Geometry: final body of the model. Coordinates: model frame, mm. A direction names the side the tool comes from. Give positions to 0.01 mm unless a question says otherwise; leave off trailing zeros. Write each loop counter-clockwise with the first axis right and the second up, starting at its lowest first coordinate (ties: lowest second). Pieces come first, ordered by that corner, then holes. Notation, with made-up numbers: (-12.5, -31) - (37.5, -31) arc R16 ccw to (37.5, -16) - close; hole circle Ø6 at (26, 14). An arc over 180 degrees is marked (long way). One line per question, with ' | ' between items. Start each with the question number.
```python
from build123d import *

# Parameters (mm, degrees)
SKETCH1_R               = 29.86111111
BOSS_EXTRUDE1_DEPTH     = 1
SKETCH2_R               = 27.5
BOSS_EXTRUDE2_DEPTH     = 9
CUT_EXTRUDE1_DEPTH      = 44.639109907
CUT_EXTRUDE1_DEPTH_BACK = 44.639109907
SKETCH3_R               = 1.25


with BuildPart() as part:
    # Sketch1 → Boss-Extrude1 (new, symmetric)
    with BuildSketch(Plane(origin=(0, 0, 0), x_dir=(1, 0, 0), z_dir=(0, 1, 0))):
        with Locations(Location((0, 0, 0), (0, 0, 270))):
            Circle(SKETCH1_R)
    extrude(amount=BOSS_EXTRUDE1_DEPTH, both=True)

    # Sketch2 → Boss-Extrude2 (add)
    with BuildSketch(Plane(origin=(0, 1, 0), x_dir=(1, 0, 0), z_dir=(0, 1, 0))):
        with Locations(Location((0, 0, 0), (0, 0, 270))):
            Circle(SKETCH2_R)
    extrude(amount=BOSS_EXTRUDE2_DEPTH)

    # Sketch3 → Cut-Extrude1 (cut, two sides: drawn at the far end of the back side and taken through both)
    with BuildSketch(Plane.XZ.offset(1).offset(-CUT_EXTRUDE1_DEPTH_BACK)):
        with Locations(Location((23.000954051, -5.917652637, 0), (0, 0, 270))):
            Circle(SKETCH3_R)
        with Locations(Location((23.514698299, 3.334885892, 0), (0, 0, 270))):
            Circle(SKETCH3_R)
        with Locations(Location((20.448542892, 12.079718275, 0), (0, 0, 270))):
            Circle(SKETCH3_R)
        with Locations(Location((14.269282196, 18.985523054, 0), (0, 0, 270))):
            Circle(SKETCH3_R)
        with Locations(Location((18.985523054, -14.269282196, 0), (0, 0, 270))):
            Circle(SKETCH3_R)
        with Locations(Location((5.917652637, 23.000954051, 0), (0, 0, 270))):
            Circle(SKETCH3_R)
        with Locations(Location((-3.334885892, 23.514698299, 0), (0, 0, 270))):
            Circle(SKETCH3_R)
        with Locations(Location((-12.079718275, 20.448542892, 0), (0, 0, 270))):
            Circle(SKETCH3_R)
        with Locations(Location((-18.985523054, 14.269282196, 0), (0, 0, 270))):
            Circle(SKETCH3_R)
        with Locations(Location((-23.000954051, 5.917652637, 0), (0, 0, 270))):
            Circle(SKETCH3_R)
        with Locations(Location((-23.514698299, -3.334885892, 0), (0, 0, 270))):
            Circle(SKETCH3_R)
        with Locations(Location((12.079718275, -20.448542892, 0), (0, 0, 270))):
            Circle(SKETCH3_R)
        with Locations(Location((3.334885892, -23.514698299, 0), (0, 0, 270))):
            Circle(SKETCH3_R)
        with Locations(Location((-5.917652637, -23.000954051, 0), (0, 0, 270))):
            Circle(SKETCH3_R)
        with Locations(Location((-14.269282196, -18.985523054, 0), (0, 0, 270))):
            Circle(SKETCH3_R)
        with Locations(Location((-20.448542892, -12.079718275, 0), (0, 0, 270))):
            Circle(SKETCH3_R)
    extrude(amount=CUT_EXTRUDE1_DEPTH + CUT_EXTRUDE1_DEPTH_BACK, mode=Mode.SUBTRACT)


solid = part.part
```
1) Section A-A, the plane x = 0. Output: boundary loops of the cut face in (y, z), plus the area to 3 significant figures.
2) Line query: L1, parallel to X at y = 5.25, z = 22.5; L2, parallel to Y at x = 20, z = -19; L3, parallel to Z at x = 19.5, y = 9. Output: solid intervals per line, ascending.
3) Section B-B, the plane z = 5.5. Output: boundary loops of the cut face in (x, y).
4) Reachability of faces 1 (the cylindrical face through (-24.397, 5.437, 12.69)), 2 (the cylindrical face through (-3.81, 4.58, 22.36)) from +Z, -Z, +X, -X, +Y, -Y: full face, straight path, thin tool, end or side. Return the list, or none.
5) First-contact query: pin 1 Ø2 at (x, z) = (23, -5.92) entering from +Y; pin 2 Ø2 at (y, z) = (4, -7) entering from -X; pin 3 Ø6 at (x, y) = (-7.5, 8.5) entering from +Z; pin 4 Ø1 at (y, z) = (7, -19) entering from +X. Flat tips, straight axial feed; report the tip coordinate or a pass-through.
6) Section D-D, the plane z = -21. Output: boundary loops of the cut face in (x, y), plus the area to 3 significant figures.
7) Section C-C, the plane y = 5.5. Give the number of separate pieces and of enclosed holes in the cut face, plus the area to 3 significant figures.
Answer key:
1) outline: (-1, -29.86) - (1, -29.86) - (1, -27.5) - (10, -27.5) - (10, 27.5) - (1, 27.5) - (1, 29.86) - (-1, 29.86) - close | area: 614 mm^2
2) L1: -15.81 to -4.06, -2.6 to 4.77, 7.06 to 15.81 | L2: -1 to 1 | L3: -19.39 to -15.41, -13.13 to 11.27, 12.89 to 19.39
3) outline: (-29.35, -1) - (-24.18, -1) - (-24.18, 10) - (-26.94, 10) - (-26.94, 1) - (-29.35, 1) - close; (-21.82, -1) - (29.35, -1) - (29.35, 1) - (26.94, 1) - (26.94, 10) - (-21.82, 10) - close
4) face 1: +Y | face 2: +Y, -Y
5) pin 1: through | pin 2: x = -26.84 | pin 3: z = 27.13 | pin 4: x = 20.35
6) outline: (-21.23, -1) - (10.96, -1) - (10.96, 10) - (-17.76, 10) - (-17.76, 1) - (-21.23, 1) - close; (13.2, -1) - (21.23, -1) - (21.23, 1) - (17.76, 1) - (17.76, 10) - (13.2, 10) - close | area: 380 mm^2
7) separate pieces: 1 | enclosed holes: 16 | area: 2,300 mm^2
